Print and shaded views of the part. All mm, measured from the part's lowest x, y and z. Round coordinates to 2 decimals unless told otherwise and drop trailing zeros. Loops run counter-clockwise (first coordinate to the right, second up) from the corner with the lowest first, then second, coordinate; pieces in that order, holes last. Notation, with made-up numbers: (-15.5, 19) - (43.5, 19) arc R9 cw to (43.5, 31) - close; hole circle Ø1 at (46, 3.5). An arc over 180 degrees is marked (long way). Answer as a JSON object with one key per item and string values.
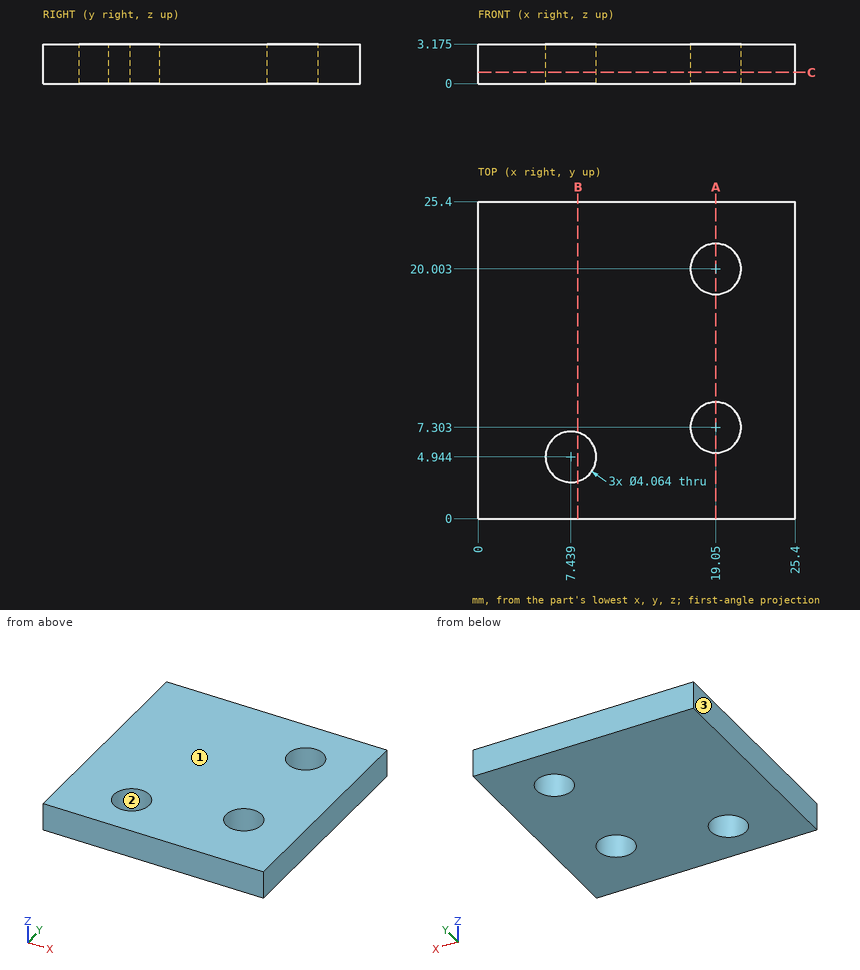
1) Slice it at C-C on z = 0.9. List the corners of the cut face in (x, y).
Values follow:
{"outline": "(0, 0) - (25.4, 0) - (25.4, 25.4) - (0, 25.4) - close; hole circle Ø4.06 at (7.44, 4.94); hole circle Ø4.06 at (19.05, 7.3); hole circle Ø4.06 at (19.05, 20)"}
2) Two-plate mould, pull along X, no slides. Class the marked faces 1, 2 and 3: pulls with the +X half, pulls with the -X half, needs draft (parallel to the pull), parting line crosses it, or undercut.
Values follow:
{"face 1": "needs draft", "face 2": "undercut", "face 3": "pulls with the -X half"}
3) Probe probe 1 along Y at (x, z) = (19.05, 0.9) (1 decimal); probe 2 along X at (y, z) = (6.5, 0.6) (1 decimal); probe 3 along X at (y, z) = (5, 1.65). List the from-to ranges inside material, lowest first.
Values follow:
{"probe 1": "0 to 5.3, 9.3 to 18, 22 to 25.4", "probe 2": "0 to 6.1, 8.7 to 17.2, 20.9 to 25.4", "probe 3": "0 to 5.41, 9.47 to 25.4"}
4) Slice it at A-A on x = 19.05. List the corners of the cut face in (y, z) (1 decimal).
Values follow:
{"outline": "(0, 0) - (5.3, 0) - (5.3, 3.2) - (0, 3.2) - close; (9.3, 0) - (18, 0) - (18, 3.2) - (9.3, 3.2) - close; (22, 0) - (25.4, 0) - (25.4, 3.2) - (22, 3.2) - close"}
5) Slice it at B-B on x = 8. List the corners of the cut face in (y, z) (1 decimal).
Values follow:
{"outline": "(0, 0) - (3, 0) - (3, 3.2) - (0, 3.2) - close; (6.9, 0) - (25.4, 0) - (25.4, 3.2) - (6.9, 3.2) - close"}
